```python
from build123d import *

# Parameters (mm, degrees)
BOSS_EXTRUDE1_DEPTH        = 4.7625
SKETCH3_R                  = 2.1
CUT_EXTRUDE1_DEPTH         = 33.69364665
SKETCH4_R                  = 4.7625
CUT_EXTRUDE2_DEPTH         = 25.4
SKETCH5_W                  = 10.115932276
SKETCH5_H                  = 25.4
BOSS_EXTRUDE2_DEPTH        = 1.5875
SKETCH6_OUTSIDE_W          = 35.822
SKETCH6_OUTSIDE_H          = 21.36
SKETCH6_OUTSIDE_R          = 4.7625
CUT_EXTRUDE3_DEPTH         = 3.175
CUT_EXTRUDE4_DEPTH         = 32.87399018
BOSS_EXTRUDE3_DEPTH        = 3.175
FILLET2_R                  = 3.175
F_2_56_TAPPED_HOLE1_REACH  = 27.374
F_2_56_TAPPED_HOLE1_BORE_R = 0.889


with BuildPart() as part:
    # Sketch2 → Boss-Extrude1 (new, symmetric)
    with BuildSketch(Plane(origin=(0, 0, 0), x_dir=(0, 0, -1), z_dir=(1, 0, 0))):
        Polygon((-4.7625, 12.7), (3, 12.7), (3, -12.7), (6.175, -12.7), (6.175, 19.05), (-4.7625, 19.05), align=None)
    extrude(amount=BOSS_EXTRUDE1_DEPTH, both=True)

    # Sketch3 → Cut-Extrude1 (cut, through all)
    with BuildSketch(Plane(origin=(0, 19.05, 0), x_dir=(1, 0, 0), z_dir=(0, 1, 0))):
        with Locations(Location((0, 0, 0), (0, 0, 270))):
            Circle(SKETCH3_R)
    extrude(amount=-CUT_EXTRUDE1_DEPTH, mode=Mode.SUBTRACT)

    # Sketch4 → Cut-Extrude2 (cut)
    with BuildSketch(Plane.XZ.offset(12.7)):
        with Locations((0, 1.0005)):
            Circle(SKETCH4_R)
    extrude(amount=-CUT_EXTRUDE2_DEPTH, mode=Mode.SUBTRACT)

    # Sketch5 → Boss-Extrude2 (add)
    with BuildSketch(Plane(origin=(0, 0, -6.175), x_dir=(-1, 0, 0), z_dir=(0, 0, -1))):
        with Locations((-7.642033862, 0)):
            Rectangle(SKETCH5_W, SKETCH5_H)
        with Locations((7.642033862, 0)):
            Rectangle(SKETCH5_W, SKETCH5_H)
    extrude(amount=-BOSS_EXTRUDE2_DEPTH)

    # Sketch6 outside → Cut-Extrude3 (cut)
    with BuildSketch(Plane(origin=(0, 19.05, 0), x_dir=(1, 0, 0), z_dir=(0, 1, 0))):
        with Locations((0, 0.706)):
            Rectangle(SKETCH6_OUTSIDE_W, SKETCH6_OUTSIDE_H)
        with Locations(Location((0, 0, 0), (0, 0, 270))):
            Circle(SKETCH6_OUTSIDE_R, mode=Mode.SUBTRACT)
    extrude(amount=-CUT_EXTRUDE3_DEPTH, mode=Mode.SUBTRACT)

    # Sketch7 → Cut-Extrude4 (cut, through all)
    with BuildSketch(Plane(origin=(0, 15.875, 0), x_dir=(1, 0, 0), z_dir=(0, 1, 0))):
        with BuildLine():
            ThreePointArc((0, -4.7625), (-3.367596045, -3.367596045), (-4.7625, 0))
            Line((-4.7625, 0), (-4.7625, -4.7625))
            Line((-4.7625, -4.7625), (0, -4.7625))
        make_face()
        with BuildLine():
            ThreePointArc((4.7625, 0), (3.367596045, -3.367596045), (0, -4.7625))
            Line((0, -4.7625), (4.7625, -4.7625))
            Line((4.7625, -4.7625), (4.7625, 0))
        make_face()
    extrude(amount=-CUT_EXTRUDE4_DEPTH, mode=Mode.SUBTRACT)

    # Sketch8 → Boss-Extrude3 (add)
    with BuildSketch(Plane(origin=(0, 15.875, 0), x_dir=(1, 0, 0), z_dir=(0, 1, 0))):
        with BuildLine():
            Line((4.7625, 6.175), (4.7625, 0))
            ThreePointArc((4.7625, 0), (0, 4.7625), (-4.7625, 0))
            Line((-4.7625, 0), (-4.7625, 6.175))
            Line((-4.7625, 6.175), (4.7625, 6.175))
        make_face()
    extrude(amount=BOSS_EXTRUDE3_DEPTH)

    # Fillet2
    fillet2_edges = [part.edges().sort_by_distance(p)[0] for p in [
        (-4.7625, 12.7, -5.38125),
        (-12.7, -12.7, -5.38125),
        (-12.7, 12.7, -5.38125),
        (4.7625, 12.7, -5.38125),
        (12.7, -12.7, -5.38125),
        (12.7, 12.7, -5.38125),
    ]]
    fillet(fillet2_edges, radius=FILLET2_R)

    # #2-56 Tapped Hole1 bore → #2-56 Tapped Hole1 (cut, up to next)
    with BuildSketch(Plane(origin=(0, 0, -6.175), x_dir=(-1, 0, 0), z_dir=(0, 0, -1)), mode=Mode.PRIVATE) as f_2_56_tapped_hole1_sk1:
        with Locations((0, 15.875)):
            Circle(F_2_56_TAPPED_HOLE1_BORE_R)
    f_2_56_tapped_hole1_tool1 = extrude(f_2_56_tapped_hole1_sk1.sketch, amount=-F_2_56_TAPPED_HOLE1_REACH, mode=Mode.PRIVATE) & part.part
    add(f_2_56_tapped_hole1_tool1.solids().sort_by_distance((0, 15.875, -6.175))[0], mode=Mode.SUBTRACT)


solid = part.part
```
Design review of the part built by this model. Coordinates are the model's own, in mm. A direction names the side the tool comes from. Coordinates: 2 decimals unless noted, no trailing zeros. Write each loop counter-clockwise with the first axis right and the second up, starting at its lowest first coordinate (ties: lowest second). Pieces come first, ordered by that corner, then holes. Notation, with made-up numbers: M 78.25,-24.5 L 116.25,-24.5 A28 ccw 116.25,1.5 Z; hole C -4.5,71.5 d3. An arc over 180 degrees is marked long. Answer as a JSON object with one key per item and string values.
Item 1: Draft analysis for pull direction Y (two halves, no side actions). For faces 1 (the cylindrical face through (0.116, 16.756, -4.069)), 2 (the flat face through (-12.7, 0, -5)), 3 (the flat face through (1.1, 19.05, -2)), state which applies: pulls with the +Y half, pulls with the -Y half, needs draft (parallel to the pull), parting line crosses it, or undercut.
Outcome:
{"face 1": "undercut", "face 2": "needs draft", "face 3": "pulls with the +Y half"}
Item 2: Add section A-A, the plane z = 1. Give the boundary of the cut face in (x, y) (3 decimals).
Outcome:
{"outline": "M -4.656,12.7 L -1.847,12.7 L -1.847,19.05 L -4.656,19.05 Z; M 1.847,12.7 L 4.656,12.7 L 4.656,19.05 L 1.847,19.05 Z"}
Item 3: Add section B-B, the plane y = -6. Give the boundary of the cut face in (x, z) (1 decimal), and give its area (3 significant figures).
Outcome:
{"outline": "M -12.7,-6.2 L 12.7,-6.2 L 12.7,-4.6 L 4.8,-4.6 L 4.8,-3 L 2.6,-3 A4.8 cw -2.6,-3 L -4.8,-3 L -4.8,-4.6 L -12.7,-4.6 Z", "area": "52.8 mm²"}
Item 4: Add section C-C, the plane z = -1.25. Give the boundary of the cut face in (x, y).
Outcome:
{"outline": "M -4.76,12.7 L -1.69,12.7 L -1.69,19.05 L -4.76,19.05 Z; M 1.69,12.7 L 4.76,12.7 L 4.76,19.05 L 1.69,19.05 Z"}
Item 5: Add section D-D, the plane z = 3. Give the boundary of the cut face in (x, y) (3 decimals).
Outcome:
{"outline": "M -3.699,12.7 L 3.699,12.7 L 3.699,19.05 L -3.699,19.05 Z"}
Item 6: Insertion check: pin 1 Ø1.7 at (x, y) = (-4, -3) entering from +Z; pin 2 Ø5.5 at (x, z) = (0, 0) entering from -Y; pin 3 Ø6 at (x, y) = (-9, 12.5) entering from +Z; pin 4 Ø2 at (x, z) = (-6, 3.5) entering from +Y. Each pin has a flat end and moves straight along its axis. Give the tip position at first contact, or say it passes through.
Outcome:
{"pin 1": "z = -3", "pin 2": "y = 12.7", "pin 3": "z = -4.59", "pin 4": "through"}
Item 7: Wall thickness on probe 1 along Z at (x, y) = (0, 17.5) (1 decimal); probe 2 along Y at (x, z) = (0, -3.4); probe 3 along Y at (x, z) = (0, -5.3): over which ranges is each line inside the solid? List them lowest first.
Outcome:
{"probe 1": "-6.2 to -2.1, 2.1 to 4.8", "probe 2": "12.7 to 14.99, 16.76 to 19.05", "probe 3": "-12.7 to 14.99, 16.76 to 19.05"}
Item 8: Machinability: for faces 4 (the flat face through (9, 12.7, -5)), 5 (the flat face through (9, -1, -4.588)), 6 (the cylindrical face through (0.631, 15.919, 2.003)), 7 (the flat face through (-9, 12.7, -5)), 8 (the flat face through (12.7, 0, -5)), which of the approach directions +Z, -Z, +X, -X, +Y, -Y give a long, thin tool a straight path to every point of the face, cutting with its end or side? Answer none if there is none.
Outcome:
{"face 4": "+Z, -Z, +X, +Y", "face 5": "+Z, +X, +Y, -Y", "face 6": "+Y, -Y", "face 7": "+Z, -Z, -X, +Y", "face 8": "+Z, -Z, +X, +Y, -Y"}
